Geometry check sheet. Reference: the model listing, model coordinates, mm. A direction names the side the tool comes from. Give positions to 0.01 mm unless a question says otherwise; leave off trailing zeros. Loops run counter-clockwise (first coordinate to the right, second up) from the corner with the lowest first, then second, coordinate; pieces in that order, holes last. Notation, with made-up numbers: (55.5, -38) -> (80.5, -38) arc R24 ccw to (80.5, -9) -> close; hole circle Ø7 at (77, -32.5). An arc over 180 degrees is marked (long way). One line per item, written item: value. Start each with the question number.
(1) Draft check along X on faces 1 (the face through (15, 15, 1)), 2 (the face through (-2.5, 8, 3)), 3 (the face through (17, 8, 0)), 4 (the face through (0.9, 0.9, 0.5)). Enter one of: pulls with the +X half, pulls with the -X half, needs draft (parallel to the pull), parting line crosses it, or undercut.
(2) Scan lines: line 1 along X through (y, z) = (0, 2.8); line 2 along Y through (x, z) = (14, 1.5); line 3 along Z through (x, y) = (34.5, 14.5). Record each from-to range of solid material in increasing order. Write a range as from..to.
(3) Sectioned sample at B-B, the plane z = 4.35. Record the cut outline in (x, y).
(4) Sectioned sample at C-C, the plane x = 33.5. Record the cut outline in (y, z).
(5) Sectioned sample at D-D, the plane y = 15.25. Record the cut outline in (x, z).
(6) Sectioned sample at A-A, the plane y = 3.25. Record the cut outline in (x, z).
(7) Gauge pin test, flat ends, axial feed: pin 1 Ø1.6 at (x, y) = (33.5, 1) entering from +Z; pin 2 Ø1.5 at (x, y) = (6, 13.5) entering from +Z. Record the tip position at first contact, or that the pin passes through.
(8) Tool access check on faces 5 (the face through (19.96, 14.71, 0.49)), 6 (the face through (27, 15.7, 2)), 7 (the face through (18, -2.5, 3)). Record the directions out of +Z, -Z, +X, -X, +Y, -Y that give a thin tool (end or side, any length) a straight path to the whole face; none if there is none.
Autodesk Inventor part; units mm, degrees
ref_plane "YZ Plane" through (0, 0, 0) normal (1, 0, 0) x (0, 1, 0)
ref_plane "XZ Plane" through (0, 0, 0) normal (0, 1, 0) x (-1, 0, 0)
ref_plane "XY Plane" through (0, 0, 0) normal (0, 0, 1) x (1, 0, 0)
sketch "Skizze1" plane through (0, 0, 0) normal (0, 0, 1) x (1, 0, 0)
  line L0 (0, 0) -> (15.6, 0) construction
  line L1 (15.6, 0) -> (15.6, 15.6) construction
  line L2 (15.6, 15.6) -> (0, 15.6) construction
  line L3 (0, 15.6) -> (0, 0) construction
  line L4 (-0.1, 15.7) -> (15.7, 15.7)
  line L5 (15.7, 15.7) -> (15.7, -0.1)
  line L6 (15.7, -0.1) -> (-0.1, -0.1)
  line L7 (-0.1, -0.1) -> (-0.1, 15.7)
  line L8 (1.9, 15.7) -> (-0.1, 13.7)
  line L9 (13.7, 15.7) -> (15.7, 13.7)
  line L10 (15.7, 1.9) -> (13.7, -0.1)
  line L11 (1.9, -0.1) -> (-0.1, 1.9)
  line L12 (-0.1, -0.1) -> (15.7, 15.7) construction
  line L13 (15.7, -0.1) -> (-0.1, 15.7) construction
  line L14 (-1.725, 17.325) -> (17.325, 17.325)
  line L15 (17.325, 17.325) -> (17.325, -1.725)
  line L16 (17.325, -1.725) -> (-1.725, -1.725)
  line L17 (-1.725, -1.725) -> (-1.725, 17.325)
  point P0 (7.8, 7.8)
  point P1 (7.8, 7.8)
  dimension "d0" = 15.6
  dimension "d1" = 15.6
  dimension "d2" = 0.1
  dimension "d3" = 2
  dimension "d4" = 2
  dimension "d5" = 2
  dimension "d6" = 2
  dimension "d7" = 2
  dimension "d8" = 2
  dimension "d9" = 2
  dimension "d10" = 2
  dimension "d11" = 9.525
extrude "Extrusion1" add sketch "Skizze1" along normal blind 1 contours L4 L8 L7 | L4 L5 L9 | L11 L6 L7 | L5 L6 L10 | L14 L15 L16 L17
sketch "Skizze2" plane through (0, 0, 1) normal (0, 0, 1) x (1, 0, 0)
  line L0 (-1.725, -1.725) -> (17.325, -1.725)
  line L1 (17.325, -1.725) -> (17.325, 17.325)
  line L2 (17.325, 17.325) -> (-1.725, 17.325)
  line L3 (-1.725, 17.325) -> (-1.725, -1.725)
  line L4 (-0.1, 13.7) -> (1.9, 15.7)
  line L5 (1.9, 15.7) -> (13.7, 15.7)
  line L6 (13.7, 15.7) -> (15.7, 13.7)
  line L7 (15.7, 13.7) -> (15.7, 1.9)
  line L8 (15.7, 1.9) -> (13.7, -0.1)
  line L9 (13.7, -0.1) -> (1.9, -0.1)
  line L10 (1.9, -0.1) -> (-0.1, 1.9)
  line L11 (-0.1, 1.9) -> (-0.1, 13.7)
  line L12 (1.9, 15.7) -> (13.7, 15.7)
  line L13 (1.9, 15.7) -> (-0.1, 15.7)
  line L14 (-0.1, 15.7) -> (-0.1, 13.7)
  line L15 (-0.1, 1.9) -> (-0.1, 13.7)
  line L16 (-0.1, 1.9) -> (-0.1, -0.1)
  line L17 (-0.1, -0.1) -> (1.9, -0.1)
  line L18 (13.7, -0.1) -> (1.9, -0.1)
  line L19 (13.7, -0.1) -> (15.7, -0.1)
  line L20 (15.7, 1.9) -> (13.7, -0.1)
  line L21 (15.7, -0.1) -> (15.7, 1.9)
  line L22 (15.7, 13.7) -> (15.7, 1.9)
  line L23 (15.7, 13.7) -> (15.7, 15.7)
  line L24 (13.7, 15.7) -> (15.7, 13.7)
  line L25 (15.7, 15.7) -> (13.7, 15.7)
  point P0 (0, 0)
extrude "Extrusion2" add sketch "Skizze2" along normal blind 4
pattern_linear "Rechteckige Anordnung1" count 2 spacing 19.05 along (1, 0, 0)
sketch "Skizze3" plane through (0, 0, 5) normal (0, 0, 1) x (1, 0, 0)
  line L0 (36.375, 17.325) -> (-1.725, 17.325)
  line L1 (-1.725, 17.325) -> (-1.725, -1.725)
  line L2 (-1.725, -1.725) -> (36.375, -1.725)
  line L3 (-0.1, 15.7) -> (15.7, 15.7)
  line L4 (15.7, 15.7) -> (15.7, -0.1)
  line L5 (15.7, -0.1) -> (-0.1, -0.1)
  line L6 (-0.1, -0.1) -> (-0.1, 15.7)
  line L7 (36.375, -1.725) -> (36.375, 17.325)
  line L8 (-2.5, 18.1) -> (37.15, 18.1)
  line L9 (37.15, 18.1) -> (37.15, -2.5)
  line L10 (37.15, -2.5) -> (-2.5, -2.5)
  line L11 (-2.5, -2.5) -> (-2.5, 18.1)
  dimension "d25" = 0.775
extrude "Extrusion3" add sketch "Skizze3" against normal up to surface (5 mm away) contours L8 L9 L10 L11
equation "\"d1\" = d0"
equation "\"d2\" = clearance"
equation "\"d3\" = dLength"
equation "\"d4\" = dLength"
equation "\"d5\" = dLength"
equation "\"d6\" = dLength"
equation "\"d7\" = dLength"
equation "\"d8\" = dLength"
equation "\"d9\" = dLength"
equation "\"d10\" = dLength"
equation "\"d25\" = border"
equation "\"clearance\" = 0.1"
equation "\"dLength\" = 2"
equation "\"border\" = 0.775"
properties part number "Cherry_Switch_Alignment_Jig"
Calculated:
1. face 1: undercut
1. face 2: pulls with the -X half
1. face 3: needs draft
1. face 4: undercut
2. line 1: x = -2.5..-0.1, 15.7..18.95, 34.75..37.15
2. line 2: y = -2.5..-0.1, 15.7..18.1
2. line 3: z = 0..1
3. outline: (-2.5, -2.5) -> (37.15, -2.5) -> (37.15, 18.1) -> (-2.5, 18.1) -> close; hole (-0.1, -0.1) -> (15.7, -0.1) -> (15.7, 15.7) -> (-0.1, 15.7) -> close; hole (18.95, -0.1) -> (34.75, -0.1) -> (34.75, 15.7) -> (18.95, 15.7) -> close
4. outline: (-2.5, 0) -> (0.65, 0) -> (0.65, 1) -> (-0.1, 1) -> (-0.1, 5) -> (-2.5, 5) -> close; (14.95, 0) -> (18.1, 0) -> (18.1, 5) -> (15.7, 5) -> (15.7, 1) -> (14.95, 1) -> close
5. outline: (-2.5, 0) -> (1.45, 0) -> (1.45, 1) -> (-0.1, 1) -> (-0.1, 5) -> (-2.5, 5) -> close; (14.15, 0) -> (20.5, 0) -> (20.5, 1) -> (18.95, 1) -> (18.95, 5) -> (15.7, 5) -> (15.7, 1) -> (14.15, 1) -> close; (33.2, 0) -> (37.15, 0) -> (37.15, 5) -> (34.75, 5) -> (34.75, 1) -> (33.2, 1) -> close
6. outline: (-2.5, 0) -> (-0.1, 0) -> (-0.1, 5) -> (-2.5, 5) -> close; (15.7, 0) -> (18.95, 0) -> (18.95, 5) -> (15.7, 5) -> close; (34.75, 0) -> (37.15, 0) -> (37.15, 5) -> (34.75, 5) -> close
7. pin 1: stops at z = 1
7. pin 2: passes through
8. face 5: +Z, -Z
8. face 6: +Z
8. face 7: +Z, -Z, +X, -X, -Y
